Read the model definition and answer for the solid it produces. Units are mm, in the model's axes. Give positions to 0.01 mm unless a question says otherwise; leave off trailing zeros. Use one line per item in the form item = value.
```python
from build123d import *

# Parameters (mm, degrees)
SKETCH2_R                = 14.463803576
BOSS_EXTRUDE1_DEPTH      = 2.5
BOSS_EXTRUDE1_TAPER      = 20
SKETCH4_W                = 8
SKETCH4_H                = 8
BOSS_EXTRUDE2_DEPTH      = 3
FILLET2_R                = 2
CIRPATTERN1_COUNT        = 4
FILLET2_OF_CIRPATTERN1_R = 2


with BuildPart() as part:
    # Sketch2 → Boss-Extrude1 (new body)
    with BuildSketch(Plane(origin=(0, 0, 0), x_dir=(1, 0, 0), z_dir=(0, 1, 0))):
        Circle(SKETCH2_R)
    extrude(amount=BOSS_EXTRUDE1_DEPTH, taper=BOSS_EXTRUDE1_TAPER)

    # Fillet1
    # an asymmetric fillet: 6, 4 mm, written as the material it takes off along each edge
    with BuildSketch(Plane(origin=(0, 2.5, 0), x_dir=(1, 0, 0), z_dir=(0, 0, -1))) as fillet1_piece_1:
        with BuildLine():
            Bezier((14.262848017, 1.94787914), (13.55387799, 0), (8.624692292, 0), weights=[1, 0.819152044, 1])
            Line((8.624692292, 0), (13.55387799, 0))
            Line((13.55387799, 0), (14.262848017, 1.94787914))
        make_face()
    revolve(axis=Axis((0, 2.5, 0), (0, -1, 0)), mode=Mode.SUBTRACT)

    # Sketch4 → Boss-Extrude2 (add)
    with BuildSketch(Plane(origin=(0, 0, 0), x_dir=(1, 0, 0), z_dir=(0, 1, 0))):
        with Locations((-12.616427752, -12.616427752)):
            Rectangle(SKETCH4_W, SKETCH4_H)
    boss_extrude2 = extrude(amount=BOSS_EXTRUDE2_DEPTH)

    # Fillet2
    fillet2_edges = [part.edges().sort_by_distance(p)[0] for p in [
        (-8.616427752, 1.5, 16.616427752),
        (-16.616427752, 1.5, 8.616427752),
        (-16.616427752, 1.5, 16.616427752),
    ]]
    fillet(fillet2_edges, radius=FILLET2_R)

    # CirPattern1: Boss-Extrude2 ×4 about axis, 2 skipped
    cirpattern1_axis = Axis((0, 0, 0), (0, 1, 0))
    add([boss_extrude2.rotate(cirpattern1_axis, i * 360 / CIRPATTERN1_COUNT) for i in range(1, CIRPATTERN1_COUNT) if i not in (1, 3)])

    # Fillet2 of CirPattern1
    fillet2_of_cirpattern1_edges = [part.edges().sort_by_distance(p)[0] for p in [
        (8.616427752, 1.5, -16.616427752),
        (16.616427752, 1.5, -8.616427752),
        (16.616427752, 1.5, -16.616427752),
    ]]
    fillet(fillet2_of_cirpattern1_edges, radius=FILLET2_OF_CIRPATTERN1_R)


solid = part.part
```
Item 1: Given pin 1 Ø1 at (x, y) = (-2.5, 1.5) entering from -Z; pin 2 Ø0.9 at (x, y) = (-12, 1) entering from -Z; pin 3 Ø1.5 at (y, z) = (0.5, -10.5) entering from +X; pin 4 Ø1.5 at (y, z) = (1, 11) entering from +X, each flat-ended and moving along its own axis, determine where each tip first touches the part or whether it passes through.
Checks:
pin_1 = -13.78
pin_2 = -8.1
pin_3 = 16.62
pin_4 = 9.77
Item 2: Straight lines are drawn through the part: L1, parallel to Z at x = -13, y = 2.85; L2, parallel to X at y = 2.15, z = 12. For each, find the intervals that lie inside material, in ascending order. Write a range as from..to.
Checks:
L1 = 8.62..16.62
L2 = -16.62..-8.62
Item 3: Determine the mould class of faces 1 (the flat face through (-8.616, 2, 12)), 2 (the flat face through (12, 2, -8.616)), 3 (the cylindrical face through (9.22, 1.52, -16.05)) for opening direction Z: +Z half, -Z half, draft (parallel to the pull), parting line (faces both ways), or undercut.
Checks:
face_1 = draft
face_2 = undercut
face_3 = -Z half
